Here's the drawing with two shaded views (mm, measured from the low corner). I have some questions. A direction names the side the tool comes from. Coordinates: 2 decimals unless noted, no trailing zeros. Order: outer loops, then holes, each group sorted by start corner. A loop starts at its lowest first (then second) coordinate and runs counter-clockwise, first axis right, second up. Notation, with made-up numbers: (-7, -27) -> (39, -27) arc R8 cw to (39, -22) -> close; hole circle Ø9 at (-19, -25.5). An arc over 180 degrees is marked (long way). Answer as a JSON object with one key per item and string values. Group by question number.
(1) Which directions (+Z, -Z, +X, -X, +Y, -Y) give clear straight access to the entire face, cutting with the end or side of a thin tool? Please do the marked faces 1 and 2.
(2) I want a section at D-D, the plane z = 109. List the corners of the cut face in (x, y) for me (3 decimals).
(3) If we mould it in two halves opening along X, with no side actions, what happens to the marked faces 3, 4 and 5? For each: pulls with the +X half, pulls with the -X half, needs draft (parallel to the pull), parting line crosses it, or undercut.
(4) I want a section at A-A, the plane x = 14.25. List the corners of the cut face in (y, z) for me, plus the area to 3 significant figures.
(5) I want a section at B-B, the plane z = 149. List the corners of the cut face in (x, y) for me (3 decimals), plus the area to 3 significant figures.
(6) I want a section at C-C, the plane y = 12.5. List the corners of the cut face in (x, z) for me, plus the area to 3 significant figures.
(7) I need wall thicknesses on line 1 (X direction, y = 8.25, z = 79.5); line 2 (X direction, y = 4.5, z = 16). Which ranges of each line are inside material? Lowest first, please.
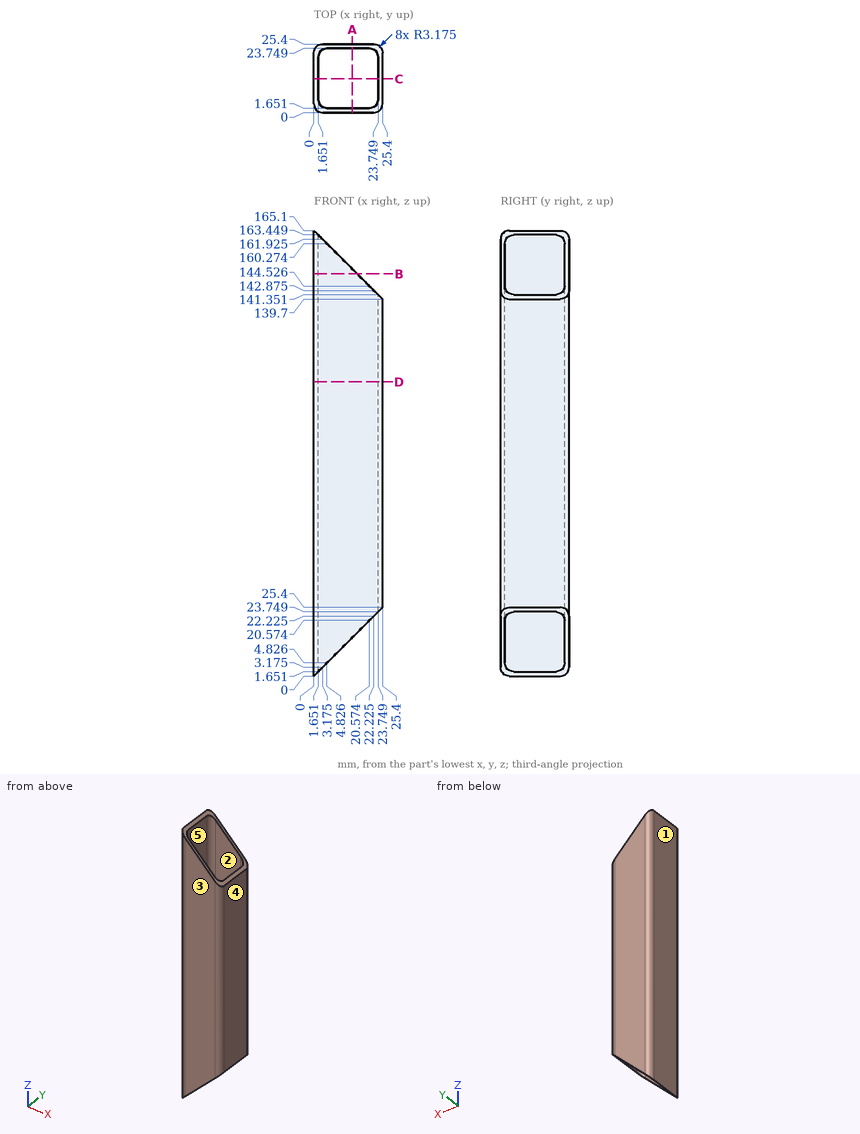
Computed values:
{
 "1": {"face 1": "+Z, -Z, -X, +Y, -Y", "face 2": "+Z, -Z"},
 "2": {"outline": "(0, 3.175) arc R3.175 ccw to (3.175, 0) -> (22.225, 0) arc R3.175 ccw to (25.4, 3.175) -> (25.4, 22.225) arc R3.175 ccw to (22.225, 25.4) -> (3.175, 25.4) arc R3.175 ccw to (0, 22.225) -> close; hole (1.651, 4.826) arc R3.175 ccw to (4.826, 1.651) -> (20.574, 1.651) arc R3.175 ccw to (23.749, 4.826) -> (23.749, 20.574) arc R3.175 ccw to (20.574, 23.749) -> (4.826, 23.749) arc R3.175 ccw to (1.651, 20.574) -> close"},
 "3": {"face 3": "needs draft", "face 4": "pulls with the +X half", "face 5": "undercut"},
 "4": {"outline": "(0, 14.25) -> (1.65, 14.25) -> (1.65, 150.85) -> (0, 150.85) -> close; (23.75, 14.25) -> (25.4, 14.25) -> (25.4, 150.85) -> (23.75, 150.85) -> close", "area": "451 mm2"},
 "5": {"outline": "(0, 3.175) arc R3.175 ccw to (3.175, 0) -> (16.1, 0) -> (16.1, 1.651) -> (4.826, 1.651) arc R3.175 cw to (1.651, 4.826) -> (1.651, 20.574) arc R3.175 cw to (4.826, 23.749) -> (16.1, 23.749) -> (16.1, 25.4) -> (3.175, 25.4) arc R3.175 ccw to (0, 22.225) -> close", "area": "89.6 mm2"},
 "6": {"outline": "(0, 0) -> (1.65, 1.65) -> (1.65, 163.45) -> (0, 165.1) -> close; (23.75, 23.75) -> (25.4, 25.4) -> (25.4, 139.7) -> (23.75, 141.35) -> close", "area": "461 mm2"},
 "7": {"line 1": "x = 0 to 1.65, 23.75 to 25.4", "line 2": "x = 0 to 1.67"}
}
